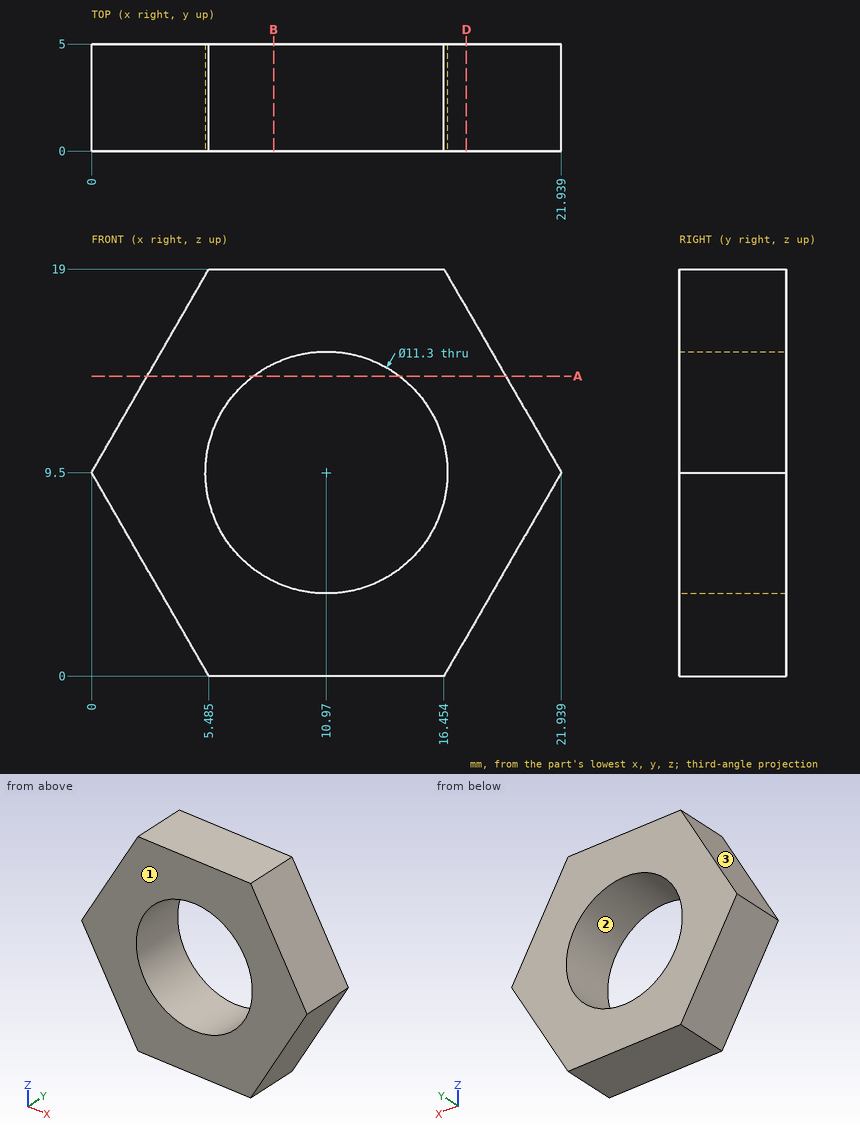
Source: three-view drawing plus pictorial views. Frame: mm from the lowest corner of the part. Coordinates: 2 decimals unless noted, no trailing zeros. Order: outer loops, then holes, each group sorted by start corner. A loop starts at its lowest first (then second) coordinate and runs counter-clockwise, first axis right, second up. Notation, with made-up numbers: M -23.75,-31.75 L -14.75,-31.75 A13 ccw -14.75,-26.75 Z; hole C -10.5,40 d7. An arc over 180 degrees is marked long. One line per question, with ' | ' between items. Start each with the question number.
Item 1: Ray query, probe 1 along Z at (x, y) = (14.5, 0.85); probe 2 along X at (y, z) = (4.25, 7.75); probe 3 along Z at (x, y) = (6.5, 1.3) (1 decimal). Return the intervals inside material, ascending. Write a range as [from, to].
Item 2: Cut plane A-A, the plane z = 14. Return the cut outline in (x, y).
Item 3: Pin query (flat end, axial travel): pin 1 Ø5 at (x, z) = (13, 7.5) entering from -Y; pin 2 Ø3 at (y, z) = (4, 3) entering from +X; pin 3 Ø2 at (y, z) = (3.5, 4.5) entering from -X. Return the tip coordinate at first contact, or that it passes through.
Item 4: Draft query along Z for the marked faces 1, 2 and 3. Return one class per face: released by +Z, released by -Z, zero draft, split by the parting line, or undercut.
Item 5: Cut plane B-B, the plane x = 8.5. Return the cut outline in (y, z).
Item 6: Cut plane D-D, the plane x = 17.5. Return the cut outline in (y, z), then the cut area to 3 significant figures.
A:
1) probe 1: z = [0, 5.09], [13.91, 19] | probe 2: x = [1.01, 5.6], [16.34, 20.93] | probe 3: z = [0, 6], [13, 19]
2) outline: M 2.6,0 L 7.55,0 L 7.55,5 L 2.6,5 Z; M 14.39,0 L 19.34,0 L 19.34,5 L 14.39,5 Z
3) pin 1: passes through | pin 2: stops at x = 19.05 | pin 3: stops at x = 2.31
4) face 1: zero draft | face 2: undercut | face 3: released by +Z
5) outline: M 0,0 L 5,0 L 5,4.42 L 0,4.42 Z; M 0,14.58 L 5,14.58 L 5,19 L 0,19 Z
6) outline: M 0,1.81 L 5,1.81 L 5,17.19 L 0,17.19 Z | area: 76.9 mm2
